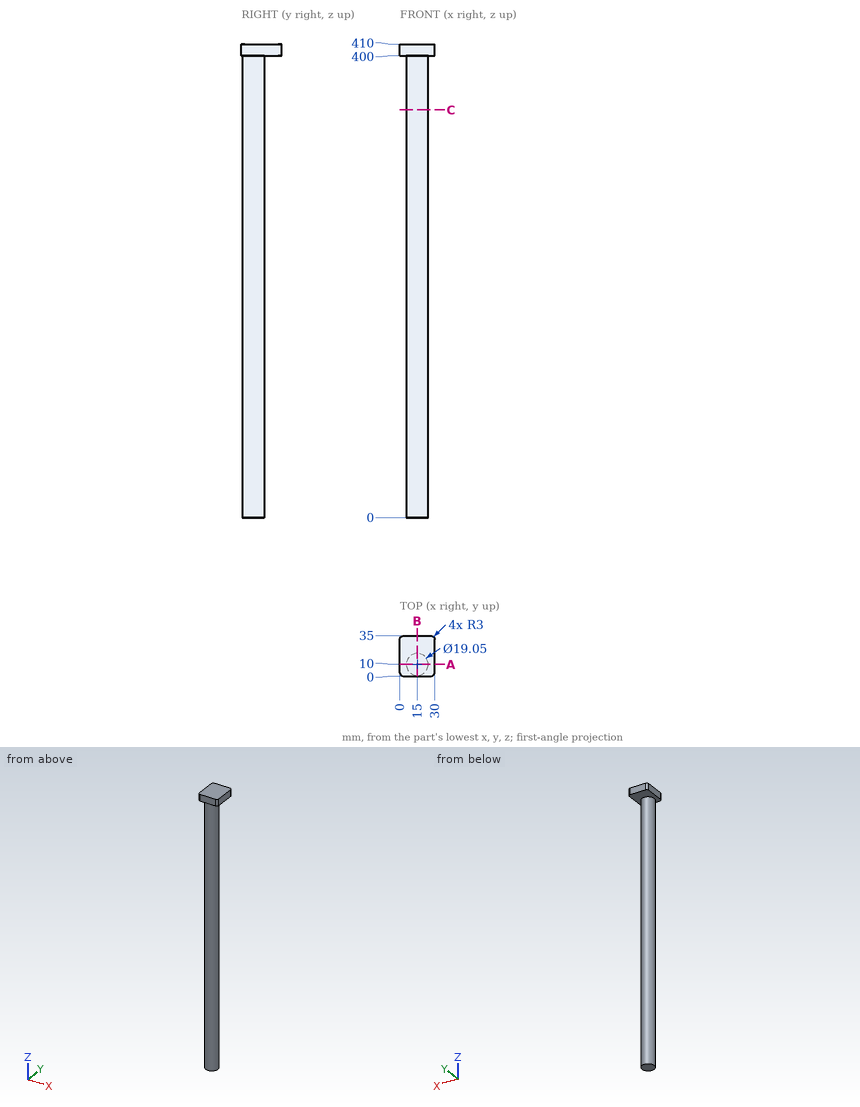
Job drawing, mm, ordinate dimensions from the low corner. One solid piece. Round coordinates to 2 decimals unless told otherwise and drop trailing zeros. Loops run counter-clockwise (first coordinate to the right, second up) from the corner with the lowest first, then second, coordinate; pieces in that order, holes last.
Item 1: Cut at B-B, the plane x = 15. Give the cut face in (y, z) (3 decimals).
Item 2: Cut at A-A, the plane y = 10. Give the cut face in (x, z) (3 decimals).
Item 3: Cut at C-C, the plane z = 353. Give the cut face in (x, y) (3 decimals), then the cut area to 3 significant figures.
Item 4: Drill centre lines: line 1 (Z direction, x = 5.75, y = 7); line 2 (Y direction, x = 16, z = 45); line 3 (X direction, y = 9.5, z = 17.5). Where is each one in solid material? Low to high.
Item 5: Drop flat-ended pins along their axis: P1, Ø12, axis at y = 14.5, z = 325, coming from the -X side (3 decimals); P2, Ø1.5, axis at y = 13, z = 251.5, coming from the -X side; P3, Ø3, axis at y = 12, z = 282.5, coming from the +X side. Give the stop position or say it passes through.
A:
1. outline: (0, 400) - (0.475, 400) - (0.475, 0) - (19.525, 0) - (19.525, 400) - (35, 400) - (35, 410) - (0, 410) - close
2. outline: (0, 400) - (5.475, 400) - (5.475, 0) - (24.525, 0) - (24.525, 400) - (30, 400) - (30, 410) - (0, 410) - close
3. outline: circle Ø19.05 at (15, 10)
3. area: 285 mm2
4. line 1: z = 400 to 410
4. line 2: y = 0.53 to 19.47
4. line 3: x = 5.49 to 24.51
5. P1: stops at x = 5.475
5. P2: stops at x = 5.74
5. P3: stops at x = 24.51
